from build123d import *

# Parameters (mm, degrees)
SKETCH1_R           = 3.5
BOSS_EXTRUDE1_DEPTH = 3
FILLET1_R           = 0.4
SKETCH2_R           = 5.5
SKETCH2_R_2         = 3.5
BOSS_EXTRUDE2_DEPTH = 1
SKETCH3_R           = 4.5
BOSS_EXTRUDE3_DEPTH = 2
SKETCH4_R           = 6
SKETCH4_R_2         = 4.5
BOSS_EXTRUDE4_DEPTH = 3
SKETCH5_R           = 4
BOSS_EXTRUDE5_DEPTH = 2
SKETCH7_R           = 3.5
BOSS_EXTRUDE6_DEPTH = 6
SKETCH8_W           = 0.5
SKETCH8_H           = 2.5
BOSS_EXTRUDE7_DEPTH = 6


with BuildPart() as part:
    # Sketch1 → Boss-Extrude1 (new body)
    with BuildSketch(Plane(origin=(0, 0, 0), x_dir=(1, 0, 0), z_dir=(0, 1, 0))):
        with Locations(Location((0, 0, 0), (0, 0, 270))):
            Circle(SKETCH1_R)
    extrude(amount=BOSS_EXTRUDE1_DEPTH)

    # Fillet1
    fillet1_edges = [part.edges().sort_by_distance(p)[0] for p in [
        (0, 3, -3.5),
    ]]
    fillet(fillet1_edges, radius=FILLET1_R)

    # Sketch2 → Boss-Extrude2 (add)
    with BuildSketch(Plane.XZ):
        with Locations(Location((0, 0, 0), (0, 0, 270))):
            Circle(SKETCH2_R)
        with Locations(Location((0, 0, 0), (0, 0, 90))):
            Circle(SKETCH2_R_2, mode=Mode.SUBTRACT)
        with Locations(Location((0, 0, 0), (0, 0, 90))):
            Circle(SKETCH2_R_2)
    extrude(amount=BOSS_EXTRUDE2_DEPTH)

    # Sketch3 → Boss-Extrude3 (add)
    with BuildSketch(Plane.XZ.offset(1)):
        with Locations(Location((0, 0, 0), (0, 0, 270))):
            Circle(SKETCH3_R)
    extrude(amount=BOSS_EXTRUDE3_DEPTH)

    # Sketch4 → Boss-Extrude4 (add)
    with BuildSketch(Plane.XZ.offset(3)):
        with Locations(Location((0, 0, 0), (0, 0, 270))):
            Circle(SKETCH4_R)
        with Locations(Location((0, 0, 0), (0, 0, 270))):
            Circle(SKETCH4_R_2, mode=Mode.SUBTRACT)
        with Locations(Location((0, 0, 0), (0, 0, 270))):
            Circle(SKETCH4_R_2)
    extrude(amount=BOSS_EXTRUDE4_DEPTH)

    # Sketch5 → Boss-Extrude5 (add)
    with BuildSketch(Plane.XZ.offset(6)):
        with Locations(Location((0, 0, 0), (0, 0, 270))):
            Circle(SKETCH5_R)
    extrude(amount=BOSS_EXTRUDE5_DEPTH)

    # Sketch7 → Boss-Extrude6 (add)
    with BuildSketch(Plane.XZ.offset(8)):
        with Locations(Location((0, 0, 0), (0, 0, 90))):
            Circle(SKETCH7_R)
    extrude(amount=BOSS_EXTRUDE6_DEPTH)

    # Sketch8 → Boss-Extrude7 (add)
    with BuildSketch(Plane.XZ.offset(14)):
        with Locations((2, 0)):
            Rectangle(SKETCH8_W, SKETCH8_H)
        with Locations((-2, 0)):
            Rectangle(SKETCH8_W, SKETCH8_H)
    extrude(amount=BOSS_EXTRUDE7_DEPTH)


solid = part.part
Read the model definition and answer for the solid it produces. Units are mm, in the model's axes. A direction names the side the tool comes from. Coordinates: 2 decimals unless noted, no trailing zeros. Write each loop counter-clockwise with the first axis right and the second up, starting at its lowest first coordinate (ties: lowest second). Pieces come first, ordered by that corner, then holes. Notation, with made-up numbers: (-1.5, -16) -> (55.5, -16) arc R13 cw to (55.5, 7) -> close; hole circle Ø1 at (53, 19). An arc over 180 degrees is marked (long way). Return JSON: item names as keys, results as strings.
(1) The part is cut by section C-C on z = -5. Give the vertices of the cut face in (x, y), then the cut area to 3 significant figures.
Answers below:
{"outline": "(-3.32, -6) -> (3.32, -6) -> (3.32, -3) -> (-3.32, -3) -> close; (-2.29, -1) -> (2.29, -1) -> (2.29, 0) -> (-2.29, 0) -> close", "area": "24.5 mm^2"}
(2) Consider line 1 along Y through (x, z) = (3, 4); line 2 along X through (y, z) = (-16.5, -0.75); line 3 along Y through (x, z) = (0, 1.5). Determine where each line is inside the solid, lowest interval first. Write a range as from..to.
Answers below:
{"line 1": "-6..-3, -1..0", "line 2": "-2.25..-1.75, 1.75..2.25", "line 3": "-14..3"}
(3) Which of the six approach directions +Z, -Z, +X, -X, +Y, -Y give full straight-line access (tool end or side, diameter ignored) to faces 1 (the flat face through (-3.92, -6, 1.42)), 2 (the flat face through (4.5, -3, 1.4)), 3 (the flat face through (1.75, -17, 0)), 4 (the cylindrical face through (-3.417, 1.282, -0.759))?
Answers below:
{"face 1": "-Y", "face 2": "none", "face 3": "+Z, -Z, -Y", "face 4": "+Y"}
(4) For a pull along Y with two mould halves and no side action, classify faces 5 (the flat face through (0, 0, -4)), 6 (the cylindrical face through (-5.37, -0.49, 1.19)), 7 (the cylindrical face through (1.352, -1.986, -4.292)) as pulls with the +Y half, pulls with the -Y half, needs draft (parallel to the pull), parting line crosses it, or undercut.
Answers below:
{"face 5": "pulls with the +Y half", "face 6": "needs draft", "face 7": "undercut"}
(5) Each of these flat-tipped pins is pushed along its axis until it touches: P1, Ø3, axis at y = -17, z = -0.5, coming from the -X side; P2, Ø2, axis at x = 2.5, y = -3.5, coming from the +Z side; P3, Ø1, axis at x = -2, y = -16.5, coming from the -Z side; P4, Ø4, axis at x = 4.5, y = -16.5, coming from the -Z side. Where does it stop, or does it pass through?
Answers below:
{"P1": "x = -2.25", "P2": "z = 5.81", "P3": "z = -1.25", "P4": "through"}
(6) The part is cut by section D-D on y = -0.25. Give the vertices of the cut face in (x, z), then the cut area to 3 significant figures.
Answers below:
{"outline": "circle Ø11 at (0, 0)", "area": "95.0 mm^2"}
(7) The part is cut by section B-B on x = 0. Give the vertices of the cut face in (y, z), then the cut area to 3 significant figures.
Answers below:
{"outline": "(-14, -3.5) -> (-8, -3.5) -> (-8, -4) -> (-6, -4) -> (-6, -6) -> (-3, -6) -> (-3, -4.5) -> (-1, -4.5) -> (-1, -5.5) -> (0, -5.5) -> (0, -3.5) -> (2.6, -3.5) arc R0.4 ccw to (3, -3.1) -> (3, 3.1) arc R0.4 ccw to (2.6, 3.5) -> (0, 3.5) -> (0, 5.5) -> (-1, 5.5) -> (-1, 4.5) -> (-3, 4.5) -> (-3, 6) -> (-6, 6) -> (-6, 4) -> (-8, 4) -> (-8, 3.5) -> (-14, 3.5) -> close", "area": "144 mm^2"}
